Could you check a few things on this model? Use its own coordinates, in mm. Face numbers are marked on the shaded views. A direction names the side the tool comes from. Round coordinates to 2 decimals unless told otherwise and drop trailing zeros. Loops run counter-clockwise (first coordinate to the right, second up) from the corner with the lowest first, then second, coordinate; pieces in that order, holes last.
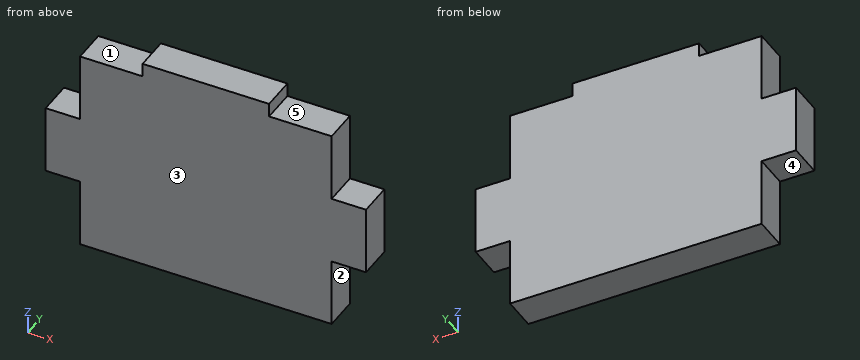
from build123d import *

# Parameters (mm, degrees)
SKETCH1_W           = 46.482
SKETCH1_H           = 38.1
BOSS_EXTRUDE1_DEPTH = 3.175
SKETCH2_W           = 23.368
SKETCH2_H           = 2.54
SKETCH2_W_2         = 6.35
SKETCH2_H_2         = 12.7
BOSS_EXTRUDE2_DEPTH = 6.35


with BuildPart() as part:
    # Sketch1 → Boss-Extrude1 (new body, symmetric)
    with BuildSketch(Plane(origin=(0, 0, 0), x_dir=(1, 0, 0), z_dir=(0, 1, 0))):
        Rectangle(SKETCH1_W, SKETCH1_H)
    extrude(amount=BOSS_EXTRUDE1_DEPTH, both=True)

    # Sketch2 → Boss-Extrude2 (add)
    with BuildSketch(Plane(origin=(0, 3.175, 0), x_dir=(1, 0, 0), z_dir=(0, 1, 0))):
        with Locations((0, -20.32)):
            Rectangle(SKETCH2_W, SKETCH2_H)
        with Locations((-26.416, 0)):
            Rectangle(SKETCH2_W_2, SKETCH2_H_2)
        with Locations((26.416, 0)):
            Rectangle(SKETCH2_W_2, SKETCH2_H_2)
    extrude(amount=-BOSS_EXTRUDE2_DEPTH)


solid = part.part
Item 1: If we section it at C-C, the plane x = 18.5: Please give me the cut outline in (y, z) (3 decimals).
Results list:
outline: (-3.175, -19.05) - (3.175, -19.05) - (3.175, 19.05) - (-3.175, 19.05) - close
Item 2: Will these pins go through, and if not, where does the flat tip stop? pin 1 (2 mm diameter, centred on y = 1, z = 21, fed in from +X); pin 2 (3 mm diameter, centred on x = 26, y = 0, fed in from -Z); pin 3 (1.9 mm diameter, centred on x = 26.5, y = -1, fed in from +Z).
Results list:
pin 1: stops at x = 11.68
pin 2: stops at z = -6.35
pin 3: stops at z = 6.35
Item 3: If we section it at B-B, the plane z = -7.5: Please give me the cut outline in (x, y) (3 decimals), then the cut area to 3 significant figures.
Results list:
outline: (-23.241, -3.175) - (23.241, -3.175) - (23.241, 3.175) - (-23.241, 3.175) - close
area: 295 mm2
Item 4: If we section it at A-A, the plane y = -0.5: Please give me the cut outline in (x, z), then the cut area to 3 significant figures.
Results list:
outline: (-29.59, -6.35) - (-23.24, -6.35) - (-23.24, -19.05) - (23.24, -19.05) - (23.24, -6.35) - (29.59, -6.35) - (29.59, 6.35) - (23.24, 6.35) - (23.24, 19.05) - (11.68, 19.05) - (11.68, 21.59) - (-11.68, 21.59) - (-11.68, 19.05) - (-23.24, 19.05) - (-23.24, 6.35) - (-29.59, 6.35) - close
area: 1,990 mm2
Item 5: For the marked faces 1, 2, 3, 4 and 5, which set-ups out of +Z, -Z, +X, -X, +Y, -Y let a thin tool reach every point of the face, with its end or its side?
Results list:
face 1: +Z, -X, +Y, -Y
face 2: -Z, +X, +Y, -Y
face 3: +Z, -Z, +X, -X, -Y
face 4: -Z, -X, +Y, -Y
face 5: +Z, +X, +Y, -Y
Item 6: If I drill on line 1 along Z through (x, y) = (-12.5, -0.75); line 2 along Z through (x, y) = (24.5, 1.75); line 3 along X through (y, z) = (1, -17), over which ranges is the centre line in solid material (lowest first)?
Results list:
line 1: z = -19.05 to 19.05
line 2: z = -6.35 to 6.35
line 3: x = -23.24 to 23.24
